from build123d import *

# Parameters (mm, degrees)
ESBO_O1_W                = 3
ESBO_O1_H                = 12
RESSALTO_EXTRUS_O1_DEPTH = 3


with BuildPart() as part:
    # Esboço1 → Ressalto-extrusão1 (new body)
    with BuildSketch(Plane.XY):
        Polygon((-31.216896784, 9.909791424), (-31.216896784, -2.090208576), (-34.216896784, -2.090208576), (-34.216896784, -14.090208576), (-31.216896784, -14.090208576), (-31.216896784, -26.090208576), (-31.216896784, -29.090208576), (-19.216896784, -29.090208576), (-19.216896784, -26.090208576), (-7.216896784, -26.090208576), (-7.216896784, -29.090208576), (4.783103216, -29.090208576), (4.783103216, -26.090208576), (16.783103216, -26.090208576), (16.783103216, -29.090208576), (28.783103216, -29.090208576), (28.783103216, -26.090208576), (28.783103216, -14.090208576), (31.783103216, -14.090208576), (31.783103216, -2.090208576), (28.783103216, -2.090208576), (28.783103216, 9.909791424), (31.783103216, 9.909791424), (31.783103216, 21.909791424), (28.783103216, 21.909791424), (28.783103216, 33.909791424), (28.783103216, 36.909791424), (16.783103216, 36.909791424), (16.783103216, 33.909791424), (4.783103216, 33.909791424), (4.783103216, 36.909791424), (-7.216896784, 36.909791424), (-7.216896784, 33.909791424), (-19.216896784, 33.909791424), (-19.216896784, 36.909791424), (-31.216896784, 36.909791424), (-31.216896784, 33.909791424), (-31.216896784, 21.909791424), (-34.216896784, 21.909791424), (-34.216896784, 9.909791424), align=None)
        with Locations((-1.216896784, -8.090208576)):
            Rectangle(ESBO_O1_W, ESBO_O1_H, mode=Mode.SUBTRACT)
        with Locations((-1.216896784, 15.909791424)):
            Rectangle(ESBO_O1_W, ESBO_O1_H, mode=Mode.SUBTRACT)
    extrude(amount=RESSALTO_EXTRUS_O1_DEPTH)


solid = part.part
The listing builds one solid part. Answer for the finished solid, in the listing's coordinates (mm). A direction names the side the tool comes from. Round coordinates to 2 decimals unless told otherwise and drop trailing zeros. Write each loop counter-clockwise with the first axis right and the second up, starting at its lowest first coordinate (ties: lowest second). Pieces come first, ordered by that corner, then holes. Notation, with made-up numbers: (68, 88.5) - (110, 88.5) arc R29 ccw to (110, 126.5) - close; hole circle Ø10 at (79.5, -28.75). An arc over 180 degrees is marked (long way). Use one line per item in the form item = value. Start each with the question number.
Item 1: A cutting plane is placed at C-C (z = 1.7). Give the number of separate pieces and of enclosed holes in the cut face, plus the area to 3 significant figures.
Item 2: Flat-ended cylindrical pins translate along their axes: pin 1 Ø3 at (x, y) = (-12.5, -12) entering from -Z; pin 2 Ø1.5 at (y, z) = (5, 2) entering from +X; pin 3 Ø1.5 at (x, z) = (-32.5, 2) entering from +Y; pin 4 Ø1.5 at (x, z) = (-16, 1.5) entering from -Y. Find the tip coordinate at first contact, or state that the pin passes through.
Item 3: A cutting plane is placed at D-D (y = -20). Write down the section's boundary in (x, z).
Item 4: A cutting plane is placed at A-A (y = -11.5). Write down the section's boundary in (x, z), plus the area to 3 significant figures.
Item 5: A cutting plane is placed at B-B (x = -15). Write down the section's boundary in (y, z), plus the area to 3 significant figures.
Item 6: Find the intervals of material crossed by line 1 (X direction, y = -3, z = 0.5); line 2 (X direction, y = 27.5, z = 2.2); line 3 (Y direction, x = 10, z = 2.4), in increasing order. Write a range as [from, to].
Item 7: A tool of negligible diameter and unlimited length cuts with its end or side. For faces 1 (the flat face through (-31.217, -21, 1)), 2 (the flat face through (-2.717, 16, 1)), 3 (the flat face through (-13, -26.09, 1)), 4 (the flat face through (-31.217, 30, 1)), 5 (the flat face through (11, 33.91, 1)), from which of +Z, -Z, +X, -X, +Y, -Y can it reach the whole face along a straight path? Write none if from no direction.
Item 8: Determine the mould class of faces 6 (the flat face through (16.783, 35, 1)), 7 (the flat face through (31.783, 16, 1)), 8 (the flat face through (-33, -14.09, 1)) for opening direction X: +X half, -X half, draft (parallel to the pull), parting line (faces both ways), or undercut.
The answers:
q1.separate_pieces = 1
q1.enclosed_holes = 2
q1.area = 3,890 mm^2
q2.pin_1 = 0
q2.pin_2 = 28.78
q2.pin_3 = 21.91
q2.pin_4 = -26.09
q3.outline = (-31.22, 0) - (28.78, 0) - (28.78, 3) - (-31.22, 3) - close
q4.outline = (-34.22, 0) - (-2.72, 0) - (-2.72, 3) - (-34.22, 3) - close; (0.28, 0) - (31.78, 0) - (31.78, 3) - (0.28, 3) - close
q4.area = 189 mm^2
q5.outline = (-26.09, 0) - (33.91, 0) - (33.91, 3) - (-26.09, 3) - close
q5.area = 180 mm^2
q6.line_1 = [-34.22, -2.72], [0.28, 31.78]
q6.line_2 = [-31.22, 28.78]
q6.line_3 = [-26.09, 33.91]
q7.face_1 = +Z, -Z, -X, -Y
q7.face_2 = +Z, -Z
q7.face_3 = +Z, -Z, -Y
q7.face_4 = +Z, -Z, -X, +Y
q7.face_5 = +Z, -Z, +Y
q8.face_6 = undercut
q8.face_7 = +X half
q8.face_8 = draft
